Input: part model. Units: mm. Frame: model coordinates. Face numbers are marked on the shaded views. A direction names the side the tool comes from. Coordinates: 2 decimals unless noted, no trailing zeros. Write each loop counter-clockwise with the first axis right and the second up, starting at its lowest first coordinate (ties: lowest second). Pieces come first, ordered by that corner, then holes. Notation, with made-up numbers: M 30.5,-13.5 L 48.5,-13.5 A7 cw 48.5,-0.5 Z; hole C -2,-24 d6. An arc over 180 degrees is marked long. Answer as a JSON object with one key per item and string values. Group by question number.
from build123d import *

# Parameters (mm, degrees)
SKETCH2_R           = 1.85
BOSS_EXTRUDE1_DEPTH = 40
SKETCH3_R           = 3
BOSS_EXTRUDE2_DEPTH = 2
SKETCH4_W           = 3.7
SKETCH4_H           = 3.7
BOSS_EXTRUDE3_DEPTH = 27


with BuildPart() as part:
    # Sketch2 → Boss-Extrude1 (new body)
    with BuildSketch(Plane(origin=(0, 0, 0), x_dir=(1, 0, 0), z_dir=(0, 1, 0))):
        with Locations(Location((0, 0, 0), (0, 0, 270))):
            Circle(SKETCH2_R)
    extrude(amount=BOSS_EXTRUDE1_DEPTH)

    # Sketch3 → Boss-Extrude2 (add)
    with BuildSketch(Plane(origin=(0, 40, 0), x_dir=(1, 0, 0), z_dir=(0, 1, 0))):
        with Locations(Location((0, 0, 0), (0, 0, 270))):
            Circle(SKETCH3_R)
    extrude(amount=BOSS_EXTRUDE2_DEPTH)

    # Sketch4 → Boss-Extrude3 (add)
    with BuildSketch(Plane(origin=(0, 42, 0), x_dir=(1, 0, 0), z_dir=(0, 1, 0))):
        Rectangle(SKETCH4_W, SKETCH4_H)
    extrude(amount=BOSS_EXTRUDE3_DEPTH)


solid = part.part
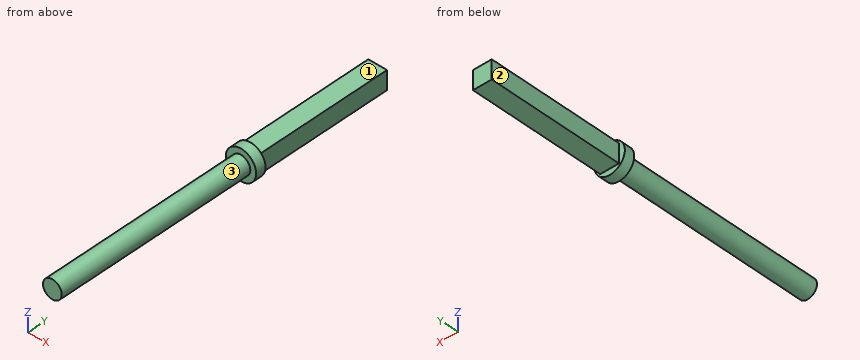
Q1. Section B-B, the plane x = 0. Return the cut outline in (y, z), and give its area (3 significant figures).
Q2. Access query for the marked faces 1, 2 and 3. Directions: +Z, -Z, +X, -X, +Y, -Y. A direction counts if a zero-diameter tool reaches every point of the face in a straight line with its end or side. Return the directions, or none.
Q3. Section A-A, the plane z = 0. Return the cut outline in (x, y).
Q4. Line query: line 1 (Y direction, x = -1.3, z = 2.4); line 2 (Y direction, x = -0.85, z = -1.7); line 3 (X direction, y = 62.5, z = -1.3). Output: solid intervals per line, ascending. Write a range as from..to.
Q5. Section D-D, the plane y = 34. Return the cut outline in (x, z), and give its area (3 significant figures).
Q6. Pin query (flat end, axial travel): pin 1 Ø1 at (y, z) = (31, -2) entering from +X; pin 2 Ø3 at (x, y) = (0, 55.5) entering from -Z; pin 3 Ø1 at (y, z) = (58.5, 0) entering from +X. Return the tip coordinate at first contact, or that it passes through.
Q7. Section C-C, the plane y = 54. Return the cut outline in (x, z), and give its area (3 significant figures).
Filled in:
{
 "1": {"outline": "M 0,-1.85 L 40,-1.85 L 40,-3 L 42,-3 L 42,-1.85 L 69,-1.85 L 69,1.85 L 42,1.85 L 42,3 L 40,3 L 40,1.85 L 0,1.85 Z", "area": "260 mm^2"},
 "2": {"face 1": "+Z, +X, -X, +Y", "face 2": "+Z, -Z, -X, +Y", "face 3": "-Y"},
 "3": {"outline": "M -3,40 L -1.85,40 L -1.85,0 L 1.85,0 L 1.85,40 L 3,40 L 3,42 L 1.85,42 L 1.85,69 L -1.85,69 L -1.85,42 L -3,42 Z"},
 "4": {"line 1": "40..42", "line 2": "40..69", "line 3": "-1.85..1.85"},
 "5": {"outline": "C 0,0 d3.7", "area": "10.8 mm^2"},
 "6": {"pin 1": "x = 1.08", "pin 2": "z = -1.85", "pin 3": "x = 1.85"},
 "7": {"outline": "M -1.85,-1.85 L 1.85,-1.85 L 1.85,1.85 L -1.85,1.85 Z", "area": "13.7 mm^2"}
}
